Geometry check sheet. Reference: the model listing, model coordinates, mm. Face numbers are marked on the shaded views. Give positions to 0.01 mm unless a question says otherwise; leave off trailing zeros. Write each loop counter-clockwise with the first axis right and the second up, starting at its lowest first coordinate (ties: lowest second). Pieces come first, ordered by that corner, then holes. Notation, with made-up numbers: (-39.5, 8) - (11.5, 8) arc R24 cw to (11.5, 47) - close; hole circle Ø9 at (31.5, 45). An arc over 180 degrees is marked (long way). Use a Markdown table: item, result.
```python
from build123d import *

# Parameters (mm, degrees)
F0_W     = 88.9
F0_H     = 88.9
F0_R     = 4.7625
F0_R_2   = 30.1625
F1_DEPTH = 6.35


with BuildPart() as f1:
    # F0 (on Top) → F1 (new body)
    with BuildSketch(Plane.XY):
        Rectangle(F0_W, F0_H)
        with Locations((-31.75, -31.75)):
            Circle(F0_R, mode=Mode.SUBTRACT)
        with Locations((31.75, -31.75)):
            Circle(F0_R, mode=Mode.SUBTRACT)
        with Locations((-31.75, 31.75)):
            Circle(F0_R, mode=Mode.SUBTRACT)
        Circle(F0_R_2, mode=Mode.SUBTRACT)
        with Locations((31.75, 31.75)):
            Circle(F0_R, mode=Mode.SUBTRACT)
    extrude(amount=-F1_DEPTH)


solid = f1.part
```
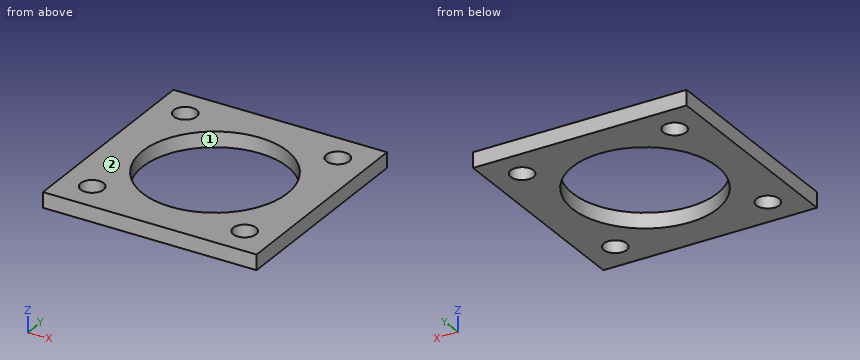
1) Section check D-D on z = -3.75. Count the separate pieces of the cut face and the enclosed holes in it, then the cut area to 3 significant figures.
Working result:
| item | result |
|---|---|
| separate pieces | 1 |
| enclosed holes | 5 |
| area | 4,760 mm² |
2) Section check B-B on y = 0. Record the boundary of the cut face in (x, z), then the cut area to 3 significant figures.
Working result:
| item | result |
|---|---|
| outline | (-44.45, -6.35) - (-30.16, -6.35) - (-30.16, 0) - (-44.45, 0) - close; (30.16, -6.35) - (44.45, -6.35) - (44.45, 0) - (30.16, 0) - close |
| area | 181 mm² |
3) Material ranges on L1, parallel to Y at x = -31.75, z = -1.75; L2, parallel to X at y = 25, z = -4.25; L3, parallel to Y at x = -2.5, z = -3.5, recorded low to high. Write a range as from..to.
Working result:
| item | result |
|---|---|
| L1 | y = -44.45..-36.51, -26.99..26.99, 36.51..44.45 |
| L2 | x = -44.45..-16.88, 16.88..44.45 |
| L3 | y = -44.45..-30.06, 30.06..44.45 |
4) Section check A-A on x = -31.75. Record the boundary of the cut face in (y, z), then the cut area to 3 significant figures.
Working result:
| item | result |
|---|---|
| outline | (-44.45, -6.35) - (-36.51, -6.35) - (-36.51, 0) - (-44.45, 0) - close; (-26.99, -6.35) - (26.99, -6.35) - (26.99, 0) - (-26.99, 0) - close; (36.51, -6.35) - (44.45, -6.35) - (44.45, 0) - (36.51, 0) - close |
| area | 444 mm² |
5) Mould release check, pull along X, two halves, no side actions. Record for the marked faces 1 and 2: pulls with the +X half, pulls with the -X half, needs draft (parallel to the pull), parting line crosses it, or undercut.
Working result:
| item | result |
|---|---|
| face 1 | undercut |
| face 2 | needs draft |
